from build123d import *

# Parameters (mm, degrees)
SALIENTE_EXTRUIR1_DEPTH    = 200
SALIENTE_EXTRUIR2_DEPTH    = 590.35443
CROQUIS6_R                 = 5
CORTAR_EXTRUIR1_DEPTH      = 591.35443038
CORTAR_EXTRUIR1_DEPTH_BACK = 10.64556962


with BuildPart() as part:
    # Croquis2 → Saliente-Extruir1 (new body)
    with BuildSketch(Plane(origin=(0, 0, 0), x_dir=(0, 0, -1), z_dir=(1, 0, 0))):
        Polygon((0, 293.35443038), (0, -306.64556962), (200, -306.64556962), (200, -296.64556962), (10, -296.64556962), (10, 293.35443038), align=None)
    extrude(amount=-SALIENTE_EXTRUIR1_DEPTH)

    # Croquis5 → Saliente-Extruir2 (add, through all)
    with BuildSketch(Plane(origin=(0, -297, 0), x_dir=(1, 0, 0), z_dir=(0, 1, 0))):
        Polygon((-100, 10), (-105, 10), (-105, 110), (-95, 110), (-95, 10), align=None)
    extrude(amount=SALIENTE_EXTRUIR2_DEPTH)

    # Croquis6 → Cortar-Extruir1 (cut, two sides)
    with BuildSketch(Plane(origin=(0, -297, 0), x_dir=(1, 0, 0), z_dir=(0, 1, 0))) as cortar_extruir1_sk:
        with Locations((-175, 175)):
            Circle(CROQUIS6_R)
        with Locations((-25, 175)):
            Circle(CROQUIS6_R)
        with Locations((-25, 25)):
            Circle(CROQUIS6_R)
        with Locations((-175, 25)):
            Circle(CROQUIS6_R)
    extrude(amount=CORTAR_EXTRUIR1_DEPTH, mode=Mode.SUBTRACT)
    extrude(cortar_extruir1_sk.sketch, amount=-CORTAR_EXTRUIR1_DEPTH_BACK, mode=Mode.SUBTRACT)


solid = part.part
Input: part model. Units: mm. Frame: model coordinates. A direction names the side the tool comes from. Coordinates: 2 decimals unless noted, no trailing zeros. Loops run counter-clockwise (first coordinate to the right, second up) from the corner with the lowest first, then second, coordinate; pieces in that order, holes last.
(1) Material intervals for probe 1 along Z at (x, y) = (-25, -304); probe 2 along Y at (x, z) = (-54.5, -160), sorted ascending.
(2) Section D-D on z = -151.5. Return the cut outline in (x, y).
(3) Section C-C on x = -68.5. Return the cut outline in (y, z).
(4) Section A-A on z = -93.5. Return the cut outline in (x, y).
(5) Set-up query: faces 1 (the face through (-100, -6, -110)), 2 (the face through (-105, -6, -59)), 3 (the face through (-95, -6, -61)). Return all of +Z, -Z, +X, -X, +Y, -Y with unobstructed straight access to the full face (end or side cutting, diameter ignored); none if empty.
(6) Section B-B on y = -110.5. Return the cut outline in (x, z).
(7) First-contact query: pin 1 Ø9 at (x, z) = (-25, -25) entering from +Y; pin 2 Ø8 at (y, z) = (28, -88) entering from -X; pin 3 Ø16 at (x, z) = (-175, -25) entering from +Y; pin 4 Ø5 at (x, y) = (-100, 9) entering from -Z. Flat tips, straight axial feed; report the tip coordinate or a pass-through.
Data:
1. probe 1: z = -200 to -180, -170 to -30, -20 to 0
1. probe 2: y = -306.65 to -296.65
2. outline: (-200, -306.65) - (0, -306.65) - (0, -296.65) - (-200, -296.65) - close
3. outline: (-306.65, -200) - (-296.65, -200) - (-296.65, -10) - (293.35, -10) - (293.35, 0) - (-306.65, 0) - close
4. outline: (-200, -306.65) - (0, -306.65) - (0, -296.65) - (-95, -296.65) - (-95, 293.35) - (-105, 293.35) - (-105, -296.65) - (-200, -296.65) - close
5. face 1: -Z, +X, -X, +Y
5. face 2: -Z, -X, +Y
5. face 3: -Z, +X, +Y
6. outline: (-200, -10) - (-105, -10) - (-105, -110) - (-95, -110) - (-95, -10) - (0, -10) - (0, 0) - (-200, 0) - close
7. pin 1: passes through
7. pin 2: stops at x = -105
7. pin 3: stops at y = -296.65
7. pin 4: stops at z = -110
